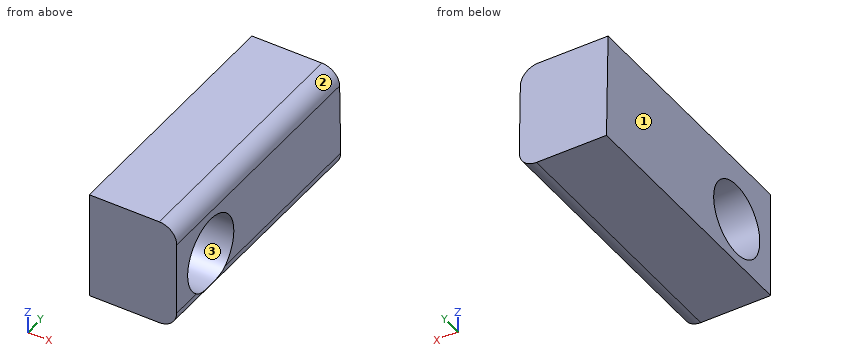
```python
from build123d import *

# Parameters (mm, degrees)
F1_R        = 10.6370455912
F2_DEPTH    = 25.4
F3_T1_DEPTH = 100.398319149
F3_T3_DEPTH = 101.1274702191


# Not quite as in the source:
# - a fillet or chamfer that OpenCascade refuses, or shapes differently, is made with other operations: its cross-section is extruded or revolved along the edge and cut away or added


with BuildPart() as f2:
    # F1 (on face) → F2 (new body)
    with BuildSketch(Plane.YZ):
        Polygon((0, 19.1946215928), (75.7274702191, 19.1946215928), (74.998319149, 50.6070703268), (0, 50.6070703268), align=None)
        with Locations((15.6783070415, 32.5921848416)):
            Circle(F1_R, mode=Mode.SUBTRACT)
    extrude(amount=F2_DEPTH)

    # F3: fillet of radius 5.08 on 2 edges, made by hand

    # F3_s2 → F3_t1 (cut)
    with BuildSketch(Plane.XZ.offset(-87.698319149)):
        with BuildLine():
            ThreePointArc((20.32, 50.6070703268), (23.9121024484, 49.1191727752), (25.4, 45.5270703268))
            Line((25.4, 45.5270703268), (25.4, 50.6070703268))
            Line((25.4, 50.6070703268), (20.32, 50.6070703268))
        make_face()
    extrude(amount=F3_T1_DEPTH, mode=Mode.SUBTRACT)

    # F3_s4 → F3_t3 (cut)
    with BuildSketch(Plane.XZ.offset(-88.4274702191)):
        with BuildLine():
            ThreePointArc((20.32, 19.1946215928), (23.9121024484, 20.6825191443), (25.4, 24.2746215928))
            Line((25.4, 24.2746215928), (25.4, 19.1946215928))
            Line((25.4, 19.1946215928), (20.32, 19.1946215928))
        make_face()
    extrude(amount=F3_T3_DEPTH, mode=Mode.SUBTRACT)


solid = f2.part
```
Here's how the part is built. I have some questions about the finished solid (model axes, mm). Face numbers are marked on the shaded views. Coordinates: 2 decimals unless noted, no trailing zeros. Order: outer loops, then holes, each group sorted by start corner. A loop starts at its lowest first (then second) coordinate and runs counter-clockwise, first axis right, second up. Notation, with made-up numbers: (55.25, -5.75) - (65.25, -5.75) arc R29 cw to (65.25, 16.25) - close; hole circle Ø7 at (28.25, 37.25). An arc over 180 degrees is marked (long way). One line per question, with ' | ' between items. Start each with the question number.
1. If we mould it in two halves opening along Z, with no side actions, what happens to the marked faces 1, 2 and 3? For each: released by +Z, released by -Z, zero draft, split by the parting line, or undercut.
2. Please list where these lines run through material, in increasing order: line 1 along Y through (x, z) = (1, 29.5); line 2 along Y through (x, z) = (14.5, 28); line 3 along X through (y, z) = (69.5, 47). Write a range as [from, to].
3. If we section it at C-C (x = 10.5): Write out the boundary of the cut face in (y, z), and give its area (3 significant figures).
4. If we section it at B-B (y = 16.5): Write out the boundary of the cut face in (x, z), and give its area (3 significant figures).
5. If we section it at A-A (z = 39): Write out the boundary of the cut face in (x, y), and give its area (3 significant figures).
6. If we section it at D-D (z = 25): Write out the boundary of the cut face in (x, y).
7. I'm going to push flat-ended pins straight in: pin 1 Ø1 at (x, z) = (8, 27) entering from +Y; pin 2 Ø4 at (x, z) = (18.5, 32) entering from +Y. Where does each tip first touch, or does it pass through?
Model answer:
1) face 1: zero draft | face 2: released by +Z | face 3: undercut
2) line 1: y = [0, 5.5], [25.86, 75.49] | line 2: y = [0, 6.08], [25.27, 75.52] | line 3: x = [0, 25.18]
3) outline: (0, 19.19) - (75.73, 19.19) - (75, 50.61) - (0, 50.61) - close; hole circle Ø21.27 at (15.68, 32.59) | area: 2,010 mm²
4) outline: (0, 19.19) - (20.32, 19.19) arc R5.08 ccw to (24.86, 21.99) - (0, 21.99) - close; (0, 43.2) - (25.4, 43.2) - (25.4, 45.53) arc R5.08 ccw to (20.32, 50.61) - (0, 50.61) - close | area: 248 mm²
5) outline: (0, 0) - (25.4, 0) - (25.4, 7.19) - (0, 7.19) - close; (0, 24.17) - (25.4, 24.17) - (25.4, 75.27) - (0, 75.27) - close | area: 1,480 mm²
6) outline: (0, 0) - (25.4, 0) - (25.4, 8.23) - (0, 8.23) - close; (0, 23.13) - (25.4, 23.13) - (25.4, 75.59) - (0, 75.59) - close
7) pin 1: stops at y = 75.56 | pin 2: stops at y = 75.48
